```python
from build123d import *

# Parameters (mm, degrees)
CROQUIS1_R              = 2.7
CROQUIS1_R_2            = 1
SALIENTE_EXTRUIR1_DEPTH = 18.8
CORTAR_EXTRUIR2_START   = -7.9
CORTAR_EXTRUIR2_DEPTH   = 7.9


with BuildPart() as part:
    # Croquis1 → Saliente-Extruir1 (new, symmetric)
    with BuildSketch(Plane.XY):
        Circle(CROQUIS1_R)
        Circle(CROQUIS1_R_2, mode=Mode.SUBTRACT)
    extrude(amount=SALIENTE_EXTRUIR1_DEPTH, both=True)

    # Croquis4 → Cortar-Extruir2 (cut)
    with BuildSketch(Plane(origin=(0, 0, -18.8), x_dir=(-1, 0, 0), z_dir=(0, 0, -1)).offset(CORTAR_EXTRUIR2_START)):
        with BuildLine():
            Line((-2.01246118, 1.8), (2.01246118, 1.8))
            ThreePointArc((2.01246118, 1.8), (0, 2.7), (-2.01246118, 1.8))
        make_face()
        with BuildLine():
            Line((-2.01246118, -1.8), (2.01246118, -1.8))
            ThreePointArc((2.01246118, -1.8), (0, -2.7), (-2.01246118, -1.8))
        make_face()
    cortar_extruir2 = extrude(amount=CORTAR_EXTRUIR2_DEPTH, mode=Mode.SUBTRACT)

    # Simetría1: Cortar-Extruir2 across plane
    add(cortar_extruir2.mirror(Plane.XY), mode=Mode.SUBTRACT)


solid = part.part
```
Input: part model. Units: mm. Frame: model coordinates. A direction names the side the tool comes from. Coordinates: 2 decimals unless noted, no trailing zeros. Write each loop counter-clockwise with the first axis right and the second up, starting at its lowest first coordinate (ties: lowest second). Pieces come first, ordered by that corner, then holes.
1) Pin query (flat end, axial travel): pin 1 Ø1 at (x, z) = (-1, 4) entering from -Y; pin 2 Ø0.7 at (x, y) = (0, 2.5) entering from +Z; pin 3 Ø2 at (x, z) = (-0.5, -16) entering from -Y. Return the tip coordinate at first contact, or that it passes through.
2) Section D-D on z = -8. Output: boundary loops of the cut face in (x, y), and give its area (3 significant figures).
3) Section A-A on x = 0. Output: boundary loops of the cut face in (y, z).
4) Mould query, pull axis X, two halves, no side actions, for faces 5 (the flat face through (0, -2, -10.9)), 6 (the cylindrical face through (0, -1, 0)), 7 (the cylindrical face through (1.246, -2.395, 0.263)). Classes: pulls with the +X half, pulls with the -X half, needs draft (parallel to the pull), parting line crosses it, or undercut.
5) Section C-C on z = 14. Output: boundary loops of the cut face in (x, y), and give its area (3 significant figures).
6) Set-up query: faces 1 (the flat face through (0, -1.8, 15)), 2 (the flat face through (0, -1.8, -15)), 3 (the flat face through (0, 2, 10.9)), 4 (the flat face through (0, 2, -10.9)). Return all of +Z, -Z, +X, -X, +Y, -Y with unobstructed straight access to the full face (end or side cutting, diameter ignored); none if empty.
7) Material intervals for line 1 along Y through (x, z) = (0, 10.5); line 2 along Y through (x, z) = (-0.65, -12); line 3 along X through (y, z) = (-0.65, 8), sorted ascending.
8) Section B-B on y = 0. Output: boundary loops of the cut face in (x, z).
Check result:
1. pin 1: stops at y = -2.65
1. pin 2: stops at z = 10.9
1. pin 3: stops at y = -1.8
2. outline: circle Ø5.4 at (0, 0); hole circle Ø2 at (0, 0)
2. area: 19.8 mm2
3. outline: (-2.7, -10.9) - (-1.8, -10.9) - (-1.8, -18.8) - (-1, -18.8) - (-1, 18.8) - (-1.8, 18.8) - (-1.8, 10.9) - (-2.7, 10.9) - close; (1, -18.8) - (1.8, -18.8) - (1.8, -10.9) - (2.7, -10.9) - (2.7, 10.9) - (1.8, 10.9) - (1.8, 18.8) - (1, 18.8) - close
4. face 5: needs draft
4. face 6: undercut
4. face 7: parting line crosses it
5. outline: (-2.01, -1.8) - (2.01, -1.8) arc R2.7 ccw to (2.01, 1.8) - (-2.01, 1.8) arc R2.7 ccw to start; hole circle Ø2 at (0, 0)
5. area: 14.7 mm2
6. face 1: +Z, +X, -X, -Y
6. face 2: -Z, +X, -X, -Y
6. face 3: +Z, +X, -X, +Y
6. face 4: -Z, +X, -X, +Y
7. line 1: y = -2.7 to -1, 1 to 2.7
7. line 2: y = -1.8 to -0.76, 0.76 to 1.8
7. line 3: x = -2.62 to -0.76, 0.76 to 2.62
8. outline: (-2.7, -18.8) - (-1, -18.8) - (-1, 18.8) - (-2.7, 18.8) - close; (1, -18.8) - (2.7, -18.8) - (2.7, 18.8) - (1, 18.8) - close
